Design review of the part built by this model. Coordinates are the model's own, in mm. Face numbers are marked on the shaded views. Coordinates: 2 decimals unless noted, no trailing zeros. Order: outer loops, then holes, each group sorted by start corner. A loop starts at its lowest first (then second) coordinate and runs counter-clockwise, first axis right, second up. Notation, with made-up numbers: (67.25, -35) -> (87.25, -35) arc R23 cw to (87.25, -4) -> close; hole circle Ø9 at (0, -24.5). An arc over 180 degrees is marked (long way). Write item = value, one per line.
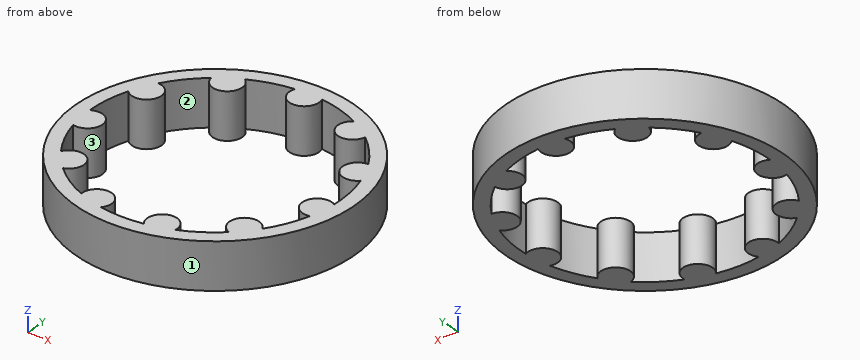
```python
from build123d import *

# Parameters (mm, degrees)
SKETCH1_R           = 30
BOSS_EXTRUDE2_DEPTH = 10


with BuildPart() as part:
    # Sketch1 → Boss-Extrude2 (new body)
    with BuildSketch(Plane.XY):
        Circle(SKETCH1_R)
        with BuildLine():
            ThreePointArc((23.097766714, 13.791586472), (20.284793496, 9.26375479), (25.548806069, 8.424558923))
            ThreePointArc((25.548806069, 8.424558923), (26.628122722, 3.828546057), (26.887372433, -0.885374634))
            ThreePointArc((26.887372433, -0.885374634), (22.073018154, -3.173620893), (26.047683788, -6.725537442))
            ThreePointArc((26.047683788, -6.725537442), (24.470870582, -11.175472139), (22.140427382, -15.28123555))
            ThreePointArc((22.140427382, -15.28123555), (16.853215508, -14.603394367), (18.276605948, -19.740323189))
            ThreePointArc((18.276605948, -19.740323189), (14.544289936, -22.631356894), (10.364053074, -24.825412151))
            ThreePointArc((10.364053074, -24.825412151), (6.282636018, -21.396693312), (4.702834857, -26.487695802))
            ThreePointArc((4.702834857, -26.487695802), (0, -26.90194574), (-4.702834857, -26.487695802))
            ThreePointArc((-4.702834857, -26.487695802), (-6.282636018, -21.396693312), (-10.364053074, -24.825412151))
            ThreePointArc((-10.364053074, -24.825412151), (-14.544289936, -22.631356894), (-18.276605948, -19.740323189))
            ThreePointArc((-18.276605948, -19.740323189), (-16.853215508, -14.603394367), (-22.140427382, -15.28123555))
            ThreePointArc((-22.140427382, -15.28123555), (-24.470870582, -11.175472139), (-26.047683788, -6.725537442))
            ThreePointArc((-26.047683788, -6.725537442), (-22.073018154, -3.173620893), (-26.887372433, -0.885374634))
            ThreePointArc((-26.887372433, -0.885374634), (-26.628122722, 3.828546057), (-25.548806069, 8.424558923))
            ThreePointArc((-25.548806069, 8.424558923), (-20.284793496, 9.26375479), (-23.097766714, 13.791586472))
            ThreePointArc((-23.097766714, 13.791586472), (-20.331134042, 17.617027932), (-16.938362942, 20.899917355))
            ThreePointArc((-16.938362942, 20.899917355), (-12.056290229, 18.759953782), (-11.974783264, 24.089816321))
            ThreePointArc((-11.974783264, 24.089816321), (-7.579153957, 25.812227914), (-2.950109262, 26.739699698))
            ThreePointArc((-2.950109262, 26.739699698), (0, 22.3), (2.950109262, 26.739699698))
            ThreePointArc((2.950109262, 26.739699698), (7.579153957, 25.812227914), (11.974783264, 24.089816321))
            ThreePointArc((11.974783264, 24.089816321), (12.056290229, 18.759953782), (16.938362942, 20.899917355))
            ThreePointArc((16.938362942, 20.899917355), (20.331134042, 17.617027932), (23.097766714, 13.791586472))
        make_face(mode=Mode.SUBTRACT)
    extrude(amount=BOSS_EXTRUDE2_DEPTH)


solid = part.part
```
(1) Insertion check: pin 1 (6 mm diameter, centred on y = 12.5, z = 8, fed in from -X); pin 2 (6 mm diameter, centred on x = 1, z = 2.5, fed in from +Y); pin 3 (1 mm diameter, centred on y = -11, z = 8.5, fed in from -X). Each pin has a flat end and moves straight along its axis. Give the tip position at first contact, or say it passes through.
Report:
pin_1 = -28.46
pin_2 = 30
pin_3 = -28.1
(2) For L1, parallel to Y at x = 16.5, z = 4.75; L2, parallel to Y at x = -11.5, z = 2.5; L3, parallel to Y at x = 23, z = 1.5, list the stretches that pass through material, from the lowest coordinate up.
Report:
L1 = -25.05 to -21.25, -18.3 to -15.1, 19.76 to 25.05
L2 = -27.71 to -24.32, 19.21 to 23.69, 24.32 to 27.71
L3 = -19.26 to -13.95, -5.91 to -1.34, 7.4 to 13.79, 13.95 to 19.26
(3) The part is to be moulded in two halves that separate along Y. For the marked faces 1, 2 and 3, say which applies: released by +Y, released by -Y, zero draft, split by the parting line, or undercut.
Report:
face_1 = split by the parting line
face_2 = undercut
face_3 = undercut
(4) We need section A-A (z = 4.25). Write out the cut boundary in (x, y), and give its area (3 significant figures).
Report:
outline = circle Ø60 at (0, 0); hole (-26.89, -0.89) arc R3.2 cw (long way) to (-26.05, -6.73) arc R26.9 ccw to (-22.14, -15.28) arc R3.2 cw (long way) to (-18.28, -19.74) arc R26.9 ccw to (-10.36, -24.83) arc R3.2 cw (long way) to (-4.7, -26.49) arc R26.9 ccw to (4.7, -26.49) arc R3.2 cw (long way) to (10.36, -24.83) arc R26.9 ccw to (18.28, -19.74) arc R3.2 cw (long way) to (22.14, -15.28) arc R26.9 ccw to (26.05, -6.73) arc R3.2 cw (long way) to (26.89, -0.89) arc R26.9 ccw to (25.55, 8.42) arc R3.2 cw (long way) to (23.1, 13.79) arc R26.9 ccw to (16.94, 20.9) arc R3.2 cw (long way) to (11.97, 24.09) arc R26.9 ccw to (2.95, 26.74) arc R3.2 cw (long way) to (-2.95, 26.74) arc R26.9 ccw to (-11.97, 24.09) arc R3.2 cw (long way) to (-16.94, 20.9) arc R26.9 ccw to (-23.1, 13.79) arc R3.2 cw (long way) to (-25.55, 8.42) arc R26.9 ccw to start
area = 823 mm²
(5) We need section B-B (x = 13.5). Write out the cut boundary in (y, z), and give its area (3 significant figures).
Report:
outline = (-26.79, 0) -> (-23.27, 0) -> (-23.27, 10) -> (-26.79, 10) -> close; (18.26, 0) -> (26.79, 0) -> (26.79, 10) -> (18.26, 10) -> close
area = 120 mm²
(6) We need section C-C (y = 25.5). Write out the cut boundary in (x, z), and give its area (3 significant figures).
Report:
outline = (-15.8, 0) -> (-8.57, 0) -> (-8.57, 10) -> (-15.8, 10) -> close; (-3.2, 0) -> (3.2, 0) -> (3.2, 10) -> (-3.2, 10) -> close; (8.57, 0) -> (15.8, 0) -> (15.8, 10) -> (8.57, 10) -> close
area = 209 mm²
(7) We need section D-D (x = -7.5). Write out the cut boundary in (y, z).
Report:
outline = (-29.05, 0) -> (-21.28, 0) -> (-21.28, 10) -> (-29.05, 10) -> close; (25.84, 0) -> (29.05, 0) -> (29.05, 10) -> (25.84, 10) -> close
